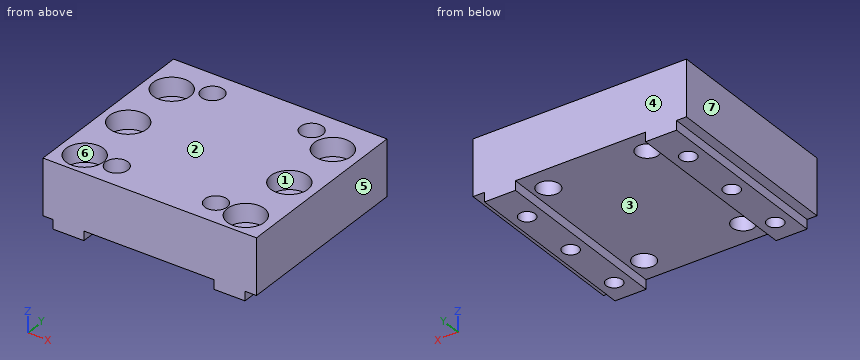
```python
from build123d import *

# Parameters (mm, degrees)
SKETCH_1_W           = 70
SKETCH_1_H           = 30
EXTRUDE_1_DEPTH      = 9
SKETCH_2_W           = 112.1
SKETCH_2_H           = 30
EXTRUDE_2_DEPTH      = 8
SKETCH_3_W           = 42.6
SKETCH_3_H           = 30
EXTRUDE_3_DEPTH      = 8
SKETCH_5_W           = 18.5
SKETCH_5_H           = 30
SKETCH_5_R           = 2
EXTRUDE_4_DEPTH      = 5.5
SKETCH_11_R          = 2
CUT_EXTRUDE_4_DEPTH  = 8
SKETCH_12_R          = 1.8
CUT_EXTRUDE_6_DEPTH  = 8
SKETCH_13_R          = 2
CUT_EXTRUDE_7_DEPTH  = 8
SKETCH_14_R          = 2
CUT_EXTRUDE_8_DEPTH  = 10
SKETCH_19_W          = 5
SKETCH_19_H          = 9
EXTRUDE_6_DEPTH      = 36.25
SKETCH_20_W          = 5
SKETCH_20_H          = 6.25
EXTRUDE_7_DEPTH      = 9
SKETCH_21_R          = 1.3
CUT_EXTRUDE_10_DEPTH = 9
SKETCH_25_W          = 5
SKETCH_25_H          = 1.5
EXTRUDE_8_DEPTH      = 42.5
SKETCH_26_R          = 1.3
CUT_EXTRUDE_14_DEPTH = 1.5
SKETCH_27_W          = 5
SKETCH_27_H          = 6.25
CUT_EXTRUDE_15_DEPTH = 11
SKETCH_28_R          = 3
CUT_EXTRUDE_16_DEPTH = 3
SKETCH_29_W          = 8
SKETCH_29_H          = 103.1
SKETCH_29_W_2        = 10.5
SKETCH_29_H_2        = 5.5
CUT_EXTRUDE_17_DEPTH = 30
SKETCH_30_R          = 1.8
CUT_EXTRUDE_18_DEPTH = 10
SKETCH_31_R          = 3.6
CUT_EXTRUDE_19_DEPTH = 3
SKETCH_32_R          = 1.8
CUT_EXTRUDE_20_DEPTH = 10
SKETCH_33_R          = 3.6
CUT_EXTRUDE_21_DEPTH = 3
CUT_EXTRUDE_22_REACH = 86.054
SKETCH_35_R          = 1.8
SKETCH_36_W          = 7.55
SKETCH_36_H          = 30
CUT_EXTRUDE_23_DEPTH = 10
SKETCH_37_W          = 18
SKETCH_37_H          = 30
SKETCH_37_W_2        = 26
CUT_EXTRUDE_24_DEPTH = 10


with BuildPart() as part:
    # 草圖1 → 填料-伸長1 (new body)
    with BuildSketch(Plane.XY):
        with Locations((35, 15)):
            Rectangle(SKETCH_1_W, SKETCH_1_H)
    extrude(amount=EXTRUDE_1_DEPTH)

    # 草圖2 → 填料-伸長2 (add)
    with BuildSketch(Plane.ZY):
        with Locations((-47.05, 15)):
            Rectangle(SKETCH_2_W, SKETCH_2_H)
    extrude(amount=EXTRUDE_2_DEPTH)

    # 草圖3 → 填料-伸長3 (add)
    with BuildSketch(Plane(origin=(70, 0, 0), x_dir=(0, 0, -1), z_dir=(1, 0, 0))):
        with Locations((12.3, 15)):
            Rectangle(SKETCH_3_W, SKETCH_3_H)
    extrude(amount=EXTRUDE_3_DEPTH)

    # 草圖5 → 填料-伸長4 (add)
    with BuildSketch(Plane(origin=(0, 0, -33.6), x_dir=(-1, 0, 0), z_dir=(0, 0, -1))):
        with Locations((-68.75, 15)):
            Rectangle(SKETCH_5_W, SKETCH_5_H)
        with Locations(Location((-65.75, 26, 0), (0, 0, 90))):
            Circle(SKETCH_5_R, mode=Mode.SUBTRACT)
        with Locations(Location((-65.75, 18, 0), (0, 0, 90))):
            Circle(SKETCH_5_R, mode=Mode.SUBTRACT)
        with Locations(Location((-65.75, 10, 0), (0, 0, 90))):
            Circle(SKETCH_5_R, mode=Mode.SUBTRACT)
    extrude(amount=EXTRUDE_4_DEPTH)

    # 草圖11 → 除料-伸長4 (cut)
    with BuildSketch(Plane.ZY.offset(8)):
        with Locations((-23, 23)):
            Circle(SKETCH_11_R)
        with Locations((-23, 15)):
            Circle(SKETCH_11_R)
        with Locations((-23, 7)):
            Circle(SKETCH_11_R)
        with Locations((-15, 23)):
            Circle(SKETCH_11_R)
        with Locations((-15, 15)):
            Circle(SKETCH_11_R)
        with Locations((-15, 7)):
            Circle(SKETCH_11_R)
        with Locations((-7, 23)):
            Circle(SKETCH_11_R)
        with Locations((-7, 15)):
            Circle(SKETCH_11_R)
        with Locations((-7, 7)):
            Circle(SKETCH_11_R)
    extrude(amount=-CUT_EXTRUDE_4_DEPTH, mode=Mode.SUBTRACT)

    # 草圖12 → 除料-伸長6 (cut)
    with BuildSketch(Plane(origin=(0, 0, -103.1), x_dir=(-1, 0, 0), z_dir=(0, 0, -1))):
        with Locations((3, 23)):
            Circle(SKETCH_12_R)
        with Locations((3, 15)):
            Circle(SKETCH_12_R)
        with Locations((3, 7)):
            Circle(SKETCH_12_R)
    extrude(amount=-CUT_EXTRUDE_6_DEPTH, mode=Mode.SUBTRACT)

    # 草圖13 → 除料-伸長7 (cut)
    with BuildSketch(Plane(origin=(78, 0, 0), x_dir=(0, 0, -1), z_dir=(1, 0, 0))):
        with Locations((9.1, 23)):
            Circle(SKETCH_13_R)
        with Locations((9.1, 15)):
            Circle(SKETCH_13_R)
        with Locations((9.1, 7)):
            Circle(SKETCH_13_R)
        with Locations((17.1, 23)):
            Circle(SKETCH_13_R)
        with Locations((17.1, 15)):
            Circle(SKETCH_13_R)
        with Locations((17.1, 7)):
            Circle(SKETCH_13_R)
        with Locations((25.1, 23)):
            Circle(SKETCH_13_R)
        with Locations((25.1, 15)):
            Circle(SKETCH_13_R)
        with Locations((25.1, 7)):
            Circle(SKETCH_13_R)
    extrude(amount=-CUT_EXTRUDE_7_DEPTH, mode=Mode.SUBTRACT)

    # 草圖14 → 除料-伸長8 (cut)
    with BuildSketch(Plane.ZY.offset(8)):
        with Locations((-85.1, 23)):
            Circle(SKETCH_14_R)
        with Locations((-85.1, 15)):
            Circle(SKETCH_14_R)
        with Locations((-85.1, 7)):
            Circle(SKETCH_14_R)
        with Locations((-77.1, 23)):
            Circle(SKETCH_14_R)
        with Locations((-77.1, 15)):
            Circle(SKETCH_14_R)
        with Locations((-77.1, 7)):
            Circle(SKETCH_14_R)
        with Locations((-69.1, 23)):
            Circle(SKETCH_14_R)
        with Locations((-69.1, 15)):
            Circle(SKETCH_14_R)
        with Locations((-69.1, 7)):
            Circle(SKETCH_14_R)
        with Locations((-61.1, 23)):
            Circle(SKETCH_14_R)
        with Locations((-61.1, 15)):
            Circle(SKETCH_14_R)
        with Locations((-61.1, 7)):
            Circle(SKETCH_14_R)
    extrude(amount=-CUT_EXTRUDE_8_DEPTH, mode=Mode.SUBTRACT)

    # 草圖19 → 填料-伸長6 (add)
    with BuildSketch(Plane(origin=(0, 30, 0), x_dir=(1, 0, 0), z_dir=(0, 1, 0))):
        with Locations((22.1, -4.5)):
            Rectangle(SKETCH_19_W, SKETCH_19_H)
        with Locations((48.1, -4.5)):
            Rectangle(SKETCH_19_W, SKETCH_19_H)
    extrude(amount=-EXTRUDE_6_DEPTH)

    # 草圖20 → 填料-伸長7 (add)
    with BuildSketch(Plane(origin=(0, 0, 0), x_dir=(-1, 0, 0), z_dir=(0, 0, -1))):
        with Locations((-48.1, 33.125)):
            Rectangle(SKETCH_20_W, SKETCH_20_H)
        with Locations((-22.1, 33.125)):
            Rectangle(SKETCH_20_W, SKETCH_20_H)
    extrude(amount=-EXTRUDE_7_DEPTH)

    # 草圖21 → 除料-伸長10 (cut)
    with BuildSketch(Plane(origin=(0, 0, 0), x_dir=(-1, 0, 0), z_dir=(0, 0, -1))):
        with Locations((-48.1, 23.75)):
            Circle(SKETCH_21_R)
        with Locations((-48.1, 13.75)):
            Circle(SKETCH_21_R)
        with Locations((-48.1, 3.75)):
            Circle(SKETCH_21_R)
        with Locations((-22.1, 23.75)):
            Circle(SKETCH_21_R)
        with Locations((-22.1, 13.75)):
            Circle(SKETCH_21_R)
        with Locations((-22.1, 3.75)):
            Circle(SKETCH_21_R)
    extrude(amount=-CUT_EXTRUDE_10_DEPTH, mode=Mode.SUBTRACT)

    # 草圖25 → 填料-伸長8 (add)
    with BuildSketch(Plane(origin=(0, 36.25, 0), x_dir=(1, 0, 0), z_dir=(0, 1, 0))):
        with Locations((22.1, 0.75)):
            Rectangle(SKETCH_25_W, SKETCH_25_H)
        with Locations((48.1, 0.75)):
            Rectangle(SKETCH_25_W, SKETCH_25_H)
    extrude(amount=-EXTRUDE_8_DEPTH)

    # 草圖26 → 除料-伸長14 (cut)
    with BuildSketch(Plane(origin=(0, 0, -1.5), x_dir=(-1, 0, 0), z_dir=(0, 0, -1))):
        with Locations((-48.1, 23.75)):
            Circle(SKETCH_26_R)
        with Locations((-48.1, 13.75)):
            Circle(SKETCH_26_R)
        with Locations((-48.1, 3.75)):
            Circle(SKETCH_26_R)
        with Locations((-22.1, 23.75)):
            Circle(SKETCH_26_R)
        with Locations((-22.1, 13.75)):
            Circle(SKETCH_26_R)
        with Locations((-22.1, 3.75)):
            Circle(SKETCH_26_R)
    extrude(amount=-CUT_EXTRUDE_14_DEPTH, mode=Mode.SUBTRACT)

    # 草圖27 → 除料-伸長15 (cut)
    with BuildSketch(Plane.XY.offset(9)):
        with Locations((22.1, 33.125)):
            Rectangle(SKETCH_27_W, SKETCH_27_H)
        with Locations((48.1, 33.125)):
            Rectangle(SKETCH_27_W, SKETCH_27_H)
        with Locations((22.1, -3.125)):
            Rectangle(SKETCH_27_W, SKETCH_27_H)
        with Locations((48.1, -3.125)):
            Rectangle(SKETCH_27_W, SKETCH_27_H)
    extrude(amount=-CUT_EXTRUDE_15_DEPTH, mode=Mode.SUBTRACT)

    # 草圖28 → 除料-伸長16 (cut)
    with BuildSketch(Plane.XY.offset(9)):
        with Locations((22.1, 23.75)):
            Circle(SKETCH_28_R)
        with Locations((22.1, 13.75)):
            Circle(SKETCH_28_R)
        with Locations((22.1, 3.75)):
            Circle(SKETCH_28_R)
        with Locations((48.1, 13.75)):
            Circle(SKETCH_28_R)
        with Locations((48.1, 3.75)):
            Circle(SKETCH_28_R)
        with Locations((48.1, 23.75)):
            Circle(SKETCH_28_R)
    extrude(amount=-CUT_EXTRUDE_16_DEPTH, mode=Mode.SUBTRACT)

    # 草圖29 → 除料-伸長17 (cut)
    with BuildSketch(Plane(origin=(0, 30, 0), x_dir=(1, 0, 0), z_dir=(0, 1, 0))):
        with Locations((-4, 51.55)):
            Rectangle(SKETCH_29_W, SKETCH_29_H)
        with Locations((64.75, 36.35)):
            Rectangle(SKETCH_29_W_2, SKETCH_29_H_2)
        Polygon((70, 33.6), (70, 0), (78, 0), (78, 39.1), (70, 39.1), align=None)
    extrude(amount=-CUT_EXTRUDE_17_DEPTH, mode=Mode.SUBTRACT)

    # 草圖30 → 除料-伸長18 (cut)
    with BuildSketch(Plane.XY.offset(9)):
        with Locations((-4, 23)):
            Circle(SKETCH_30_R)
        with Locations((-4, 15)):
            Circle(SKETCH_30_R)
        with Locations((-4, 7)):
            Circle(SKETCH_30_R)
    extrude(amount=-CUT_EXTRUDE_18_DEPTH, mode=Mode.SUBTRACT)

    # 草圖31 → 除料-伸長19 (cut)
    with BuildSketch(Plane.XY.offset(9)):
        with Locations((-4, 15)):
            Circle(SKETCH_31_R)
        with Locations((-4, 7)):
            Circle(SKETCH_31_R)
        with Locations((-4, 23)):
            Circle(SKETCH_31_R)
    extrude(amount=-CUT_EXTRUDE_19_DEPTH, mode=Mode.SUBTRACT)

    # 草圖32 → 除料-伸長20 (cut)
    with BuildSketch(Plane.XY.offset(9)):
        with Locations((65.2, 23)):
            Circle(SKETCH_32_R)
        with Locations((65.2, 15)):
            Circle(SKETCH_32_R)
        with Locations((65.2, 7)):
            Circle(SKETCH_32_R)
    extrude(amount=-CUT_EXTRUDE_20_DEPTH, mode=Mode.SUBTRACT)

    # 草圖33 → 除料-伸長21 (cut)
    with BuildSketch(Plane.XY.offset(9)):
        with Locations((65.2, 23)):
            Circle(SKETCH_33_R)
        with Locations((65.2, 15)):
            Circle(SKETCH_33_R)
        with Locations((65.2, 7)):
            Circle(SKETCH_33_R)
    extrude(amount=-CUT_EXTRUDE_21_DEPTH, mode=Mode.SUBTRACT)

    # 草圖35 → 除料-伸長22 (cut, up to next)
    with BuildSketch(Plane(origin=(0, 0, 0), x_dir=(-1, 0, 0), z_dir=(0, 0, -1)), mode=Mode.PRIVATE) as cut_extrude_22_sk1:
        with Locations((-43.1, 4)):
            Circle(SKETCH_35_R)
    cut_extrude_22_tool1 = extrude(cut_extrude_22_sk1.sketch, amount=-CUT_EXTRUDE_22_REACH, mode=Mode.PRIVATE) & part.part
    # 草圖35 → 除料-伸長22 (cut, up to next)
    with BuildSketch(Plane(origin=(0, 0, 0), x_dir=(-1, 0, 0), z_dir=(0, 0, -1)), mode=Mode.PRIVATE) as cut_extrude_22_sk2:
        with Locations((-43.1, 26)):
            Circle(SKETCH_35_R)
    cut_extrude_22_tool2 = extrude(cut_extrude_22_sk2.sketch, amount=-CUT_EXTRUDE_22_REACH, mode=Mode.PRIVATE) & part.part
    # 草圖35 → 除料-伸長22 (cut, up to next)
    with BuildSketch(Plane(origin=(0, 0, 0), x_dir=(-1, 0, 0), z_dir=(0, 0, -1)), mode=Mode.PRIVATE) as cut_extrude_22_sk3:
        with Locations((-27.1, 26)):
            Circle(SKETCH_35_R)
    cut_extrude_22_tool3 = extrude(cut_extrude_22_sk3.sketch, amount=-CUT_EXTRUDE_22_REACH, mode=Mode.PRIVATE) & part.part
    # 草圖35 → 除料-伸長22 (cut, up to next)
    with BuildSketch(Plane(origin=(0, 0, 0), x_dir=(-1, 0, 0), z_dir=(0, 0, -1)), mode=Mode.PRIVATE) as cut_extrude_22_sk4:
        with Locations((-27.1, 4)):
            Circle(SKETCH_35_R)
    cut_extrude_22_tool4 = extrude(cut_extrude_22_sk4.sketch, amount=-CUT_EXTRUDE_22_REACH, mode=Mode.PRIVATE) & part.part
    add(cut_extrude_22_tool1.solids().sort_by_distance((43.1, 4, 0))[0], mode=Mode.SUBTRACT)
    add(cut_extrude_22_tool2.solids().sort_by_distance((43.1, 26, 0))[0], mode=Mode.SUBTRACT)
    add(cut_extrude_22_tool3.solids().sort_by_distance((27.1, 26, 0))[0], mode=Mode.SUBTRACT)
    add(cut_extrude_22_tool4.solids().sort_by_distance((27.1, 4, 0))[0], mode=Mode.SUBTRACT)

    # 草圖36 → 除料-伸長23 (cut)
    with BuildSketch(Plane.XY.offset(9)):
        with Locations((74.225, 15)):
            Rectangle(SKETCH_36_W, SKETCH_36_H)
    extrude(amount=-CUT_EXTRUDE_23_DEPTH, mode=Mode.SUBTRACT)

    # 草圖37 → 除料-伸長24 (cut)
    with BuildSketch(Plane.XY.offset(9)):
        with Locations((61.45, 15)):
            Rectangle(SKETCH_37_W, SKETCH_37_H)
        with Locations((5, 15)):
            Rectangle(SKETCH_37_W_2, SKETCH_37_H)
    extrude(amount=-CUT_EXTRUDE_24_DEPTH, mode=Mode.SUBTRACT)


solid = part.part
```
The model under review builds one solid part; all positions refer to its coordinate system, in mm. Face numbers are marked on the shaded views. A direction names the side the tool comes from. Round coordinates to 2 decimals unless told otherwise and drop trailing zeros. Write each loop counter-clockwise with the first axis right and the second up, starting at its lowest first coordinate (ties: lowest second). Pieces come first, ordered by that corner, then holes. Notation, with made-up numbers: (40.5, 30.25) - (96.5, 30.25) arc R23 ccw to (96.5, 47.25) - close; hole circle Ø9 at (35, 40.5). An arc over 180 degrees is marked (long way). One line per question, with ' | ' between items.
Item 1: Add section B-B, the plane y = 23.75. Give the boundary of the cut face in (x, z).
Resolved:
outline: (18, 0) - (19.6, 0) - (19.6, -1.5) - (20.8, -1.5) - (20.8, 6) - (19.1, 6) - (19.1, 9) - (18, 9) - close; (23.4, -1.5) - (24.6, -1.5) - (24.6, 0) - (45.6, 0) - (45.6, -1.5) - (46.8, -1.5) - (46.8, 6) - (45.1, 6) - (45.1, 9) - (25.1, 9) - (25.1, 6) - (23.4, 6) - close; (49.4, -1.5) - (50.6, -1.5) - (50.6, 0) - (52.45, 0) - (52.45, 9) - (51.1, 9) - (51.1, 6) - (49.4, 6) - close
Item 2: For P1, Ø4.5, axis at x = 43.1, y = 26, coming from the -Z side; P2, Ø2, axis at x = 48.1, y = 23.75, coming from the -Z side; P3, Ø5.5, axis at x = 22.1, y = 3.75, coming from the +Z side; P4, Ø0.8, axis at y = 15.5, z = -0.5, coming from the +X side, all flat-tipped, find the tip position at first contact; note any pin that passes through.
Resolved:
P1: stops at z = 0 | P2: passes through | P3: stops at z = 6 | P4: stops at x = 50.6
Item 3: Add section A-A, the plane x = 48.1. Give the boundary of the cut face in (y, z).
Resolved:
outline: (0, -1.5) - (2.45, -1.5) - (2.45, 6) - (0.75, 6) - (0.75, 9) - (0, 9) - close; (5.05, -1.5) - (12.45, -1.5) - (12.45, 6) - (10.75, 6) - (10.75, 9) - (6.75, 9) - (6.75, 6) - (5.05, 6) - close; (15.05, -1.5) - (22.45, -1.5) - (22.45, 6) - (20.75, 6) - (20.75, 9) - (16.75, 9) - (16.75, 6) - (15.05, 6) - close; (25.05, -1.5) - (30, -1.5) - (30, 9) - (26.75, 9) - (26.75, 6) - (25.05, 6) - close
Item 4: Add section C-C, the plane x = 43.1. Give the boundary of the cut face in (y, z), then the cut area to 3 significant figures.
Resolved:
outline: (0, 0) - (2.2, 0) - (2.2, 9) - (0, 9) - close; (5.8, 0) - (24.2, 0) - (24.2, 9) - (5.8, 9) - close; (27.8, 0) - (30, 0) - (30, 9) - (27.8, 9) - close | area: 205 mm2
Item 5: The part is to be moulded in two halves that separate along X. For the marked faces 4, 5, 6 and 7, say which applies: pulls with the +X half, pulls with the -X half, needs draft (parallel to the pull), parting line crosses it, or undercut.
Resolved:
face 4: needs draft | face 5: pulls with the +X half | face 6: undercut | face 7: pulls with the -X half
Item 6: For the marked faces 1, 2 and 3, list the 3-axis set-ups (+Z, -Z, +X, -X, +Y, -Y) from which the entire face can be reached by the end or side of a thin tool; tool diameter is ignored.
Resolved:
face 1: +Z | face 2: +Z, +X, -X, +Y, -Y | face 3: -Z, +Y, -Y
Item 7: Add section D-D, the plane z = 1. State how many separate pieces and enclosed holes the cut face has, then the cut area to 3 significant figures.
Resolved:
separate pieces: 1 | enclosed holes: 10 | area: 961 mm2
Item 8: To check wall thickness, follow probe 1 along Y at (x, z) = (22.1, 7.6); probe 2 along Y at (x, z) = (48.1, 1.5); probe 3 along Y at (x, z) = (27, 2.5). State the ranges of each line that lie inside material, in increasing order.
Resolved:
probe 1: y = 0 to 0.75, 6.75 to 10.75, 16.75 to 20.75, 26.75 to 30 | probe 2: y = 0 to 2.45, 5.05 to 12.45, 15.05 to 22.45, 25.05 to 30 | probe 3: y = 0 to 2.2, 5.8 to 24.2, 27.8 to 30
